Input: part model. Units: mm. Frame: model coordinates. A direction names the side the tool comes from. Round coordinates to 2 decimals unless told otherwise and drop trailing zeros. Order: outer loops, then holes, each group sorted by start corner. A loop starts at its lowest first (then second) coordinate and runs counter-clockwise, first axis right, second up. Notation, with made-up numbers: (77, 53.5) - (110, 53.5) arc R14 ccw to (110, 80.5) - close; hole circle Ø8 at (-36, -12). An arc over 180 degrees is marked (long way). One line per item, written item: value. Start each with the question number.
Autodesk Inventor part; units mm, degrees
ref_plane "YZ Plane" through (0, 0, 0) normal (1, 0, 0) x (0, 1, 0)
ref_plane "XZ Plane" through (0, 0, 0) normal (0, 1, 0) x (-1, 0, 0)
ref_plane "XY Plane" through (0, 0, 0) normal (0, 0, 1) x (1, 0, 0)
sketch "Sketch1" plane through (0, 0, 0) normal (0, 1, 0) x (-1, 0, 0)
  line L0 (0, 0) -> (-31.75, 0)
  line L1 (-31.75, 0) -> (-31.75, 60.325)
  line L2 (-31.75, 60.325) -> (0, 60.325)
  line L3 (0, 60.325) -> (0, 0)
  line L4 (0, 60.325) -> (-25.4, 60.325)
  line L5 (-25.4, 60.325) -> (-25.4, 9.525)
  line L6 (-25.4, 9.525) -> (0, 9.525)
  line L7 (0, 9.525) -> (0, 60.325)
  dimension "d0" = 60.325
  dimension "d1" = 31.75
  dimension "d2" = 9.525
  dimension "d3" = 6.35
extrude "Extrusion1" add sketch "Sketch1" along normal blind 19.05 contours L0 L1 L2 L5 L6 L3
sketch "Sketch2" plane through (31.75, 0, 60.325) normal (1, 0, 0) x (0, 0, -1)
  line L0 (0, 0) -> (60.325, 0)
  line L1 (60.325, 0) -> (60.325, 19.05)
  line L2 (0, 19.05) -> (60.325, 19.05)
  line L3 (0, 0) -> (0, 19.05)
  point P0 (9.525, 9.525)
  dimension "d6" = 19.05
  dimension "d7" = 9.525
  dimension "d8" = 9.525
hole "Hole1" at (31.75, 9.525, 50.8) direction (-1, 0, 0) diameter 8.128 depth 10.9728 tip angle 118
sketch "Sketch3" plane through (0, 0, 0) normal (-1, 0, 0) x (0, 0, 1)
  line L0 (9.525, 0) -> (9.525, 19.05)
  line L1 (0, 19.05) -> (9.525, 19.05)
  line L2 (0, 0) -> (0, 19.05)
  line L3 (0, 0) -> (9.525, 0)
  point P0 (4.7625, 4.7625)
  point P1 (4.7625, 14.2875)
  dimension "d16" = 9.525
  dimension "d17" = 9.525
  dimension "d18" = 4.7625
  dimension "d19" = 19.05
  dimension "d20" = 4.7625
  dimension "d21" = 4.7625
hole "Hole2" at (0, 4.7625, 4.7625) at (0, 14.2875, 4.7625) direction (1, 0, 0) diameter 3.81 end through all
properties part number "PaddleCollection2.1WheelBracket" material "Nylon 6/6"
Item 1: Line query: L1, parallel to Z at x = 26, y = 6.25 (3 decimals); L2, parallel to Y at x = 29.5, z = 50.8; L3, parallel to Y at x = 10.5, z = 6.5. Output: solid intervals per line, ascending.
Item 2: Section query C-C on x = 28. Give the number of separate pieces and of enclosed holes in the cut face, and give its area (3 significant figures).
Item 3: First-contact query: pin 1 Ø2 at (x, y) = (14, 13.5) entering from -Z; pin 2 Ø5 at (y, z) = (9, 14) entering from -X. Flat tips, straight axial feed; report the tip coordinate or a pass-through.
Item 4: Pull-direction query (Z, two-part tool) for faces 3 (the face through (28.531, 11.998, 54.025)), 4 (the face through (27, 0, 21)), 5 (the face through (16, 9, 0)), 6 (the face through (13, 9, 9.525)); classes: released by +Z, released by -Z, zero draft, split by the parting line, or undercut.
Item 5: Section query D-D on z = 33. Return loops of the section in (x, y), and give its area (3 significant figures).
Item 6: Reachability of faces 1 (the face through (29, 9, 60.325)), 2 (the face through (25.4, 9, 35)) from +Z, -Z, +X, -X, +Y, -Y: full face, straight path, thin tool, end or side. Return the list, or none.
Item 7: Section query B-B on y = 8. Return loops of the section in (x, z) (3 decimals), and give its area (3 significant figures).
Item 8: Section query A-A on z = 50.8. Return loops of the section in (x, y), and give its area (3 significant figures).
Geometry results:
1. L1: z = 0 to 3.572, 5.953 to 48.394, 53.206 to 60.325
1. L2: y = 0 to 5.46, 13.59 to 19.05
1. L3: y = 0 to 3.98, 5.54 to 13.51, 15.07 to 19.05
2. separate pieces: 1
2. enclosed holes: 3
2. area: 1,070 mm^2
3. pin 1: stops at z = 0
3. pin 2: stops at x = 25.4
4. face 3: undercut
4. face 4: zero draft
4. face 5: released by -Z
4. face 6: released by +Z
5. outline: (25.4, 0) - (31.75, 0) - (31.75, 19.05) - (25.4, 19.05) - close
5. area: 121 mm^2
6. face 1: +Z, +X, -X, +Y, -Y
6. face 2: +Z, -X, +Y, -Y
7. outline: (0, 0) - (31.75, 0) - (31.75, 47.033) - (25.4, 47.033) - (25.4, 9.525) - (0, 9.525) - close; (25.4, 54.567) - (31.75, 54.567) - (31.75, 60.325) - (25.4, 60.325) - close
7. area: 577 mm^2
8. outline: (25.4, 0) - (31.75, 0) - (31.75, 5.46) - (25.4, 5.46) - close; (25.4, 13.59) - (31.75, 13.59) - (31.75, 19.05) - (25.4, 19.05) - close
8. area: 69.4 mm^2
